Part print with two shaded views. Sizes in mm from the minimum x, y, z corner. A direction names the side the tool comes from. Round coordinates to 2 decimals unless told otherwise and drop trailing zeros. Write each loop counter-clockwise with the first axis right and the second up, starting at its lowest first coordinate (ties: lowest second). Pieces come first, ordered by that corner, then holes. Notation, with made-up numbers: (67, 36) -> (97, 36) arc R15 ccw to (97, 51) -> close; hole circle Ø10 at (74, 75). An arc over 180 degrees is marked (long way). Answer as CSV lines item,"result".
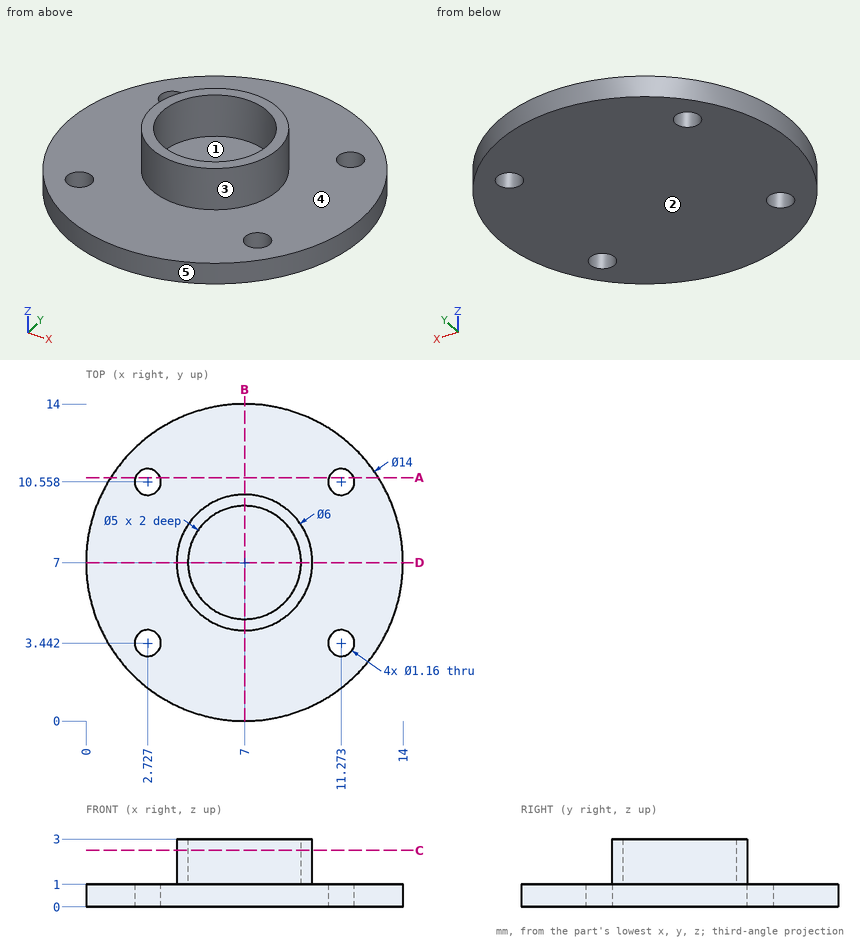
1. Cut at B-B, the plane x = 7. Write the cut outline in (y, z).
Results found:
outline,"(0, 0) -> (14, 0) -> (14, 1) -> (10, 1) -> (10, 3) -> (9.5, 3) -> (9.5, 1) -> (4.5, 1) -> (4.5, 3) -> (4, 3) -> (4, 1) -> (0, 1) -> close"
2. Mould opens along X. For the marked faces 1, 2 and 3 say: +X half, -X half, draft (parallel to the pull), parting line (faces both ways), or undercut.
Results found:
face 1,"undercut"
face 2,"draft"
face 3,"parting line"
3. Probe line 1 along Z through (x, y) = (8.75, 1.75); line 2 along Y through (x, z) = (7.5, 1.7); line 3 along Y through (x, z) = (7, 2.45). List the from-to ranges inside material, lowest first.
Results found:
line 1,"z = 0 to 1"
line 2,"y = 4.04 to 4.55, 9.45 to 9.96"
line 3,"y = 4 to 4.5, 9.5 to 10"
4. Cut at C-C, the plane z = 2.5. Write the cut outline in (x, y).
Results found:
outline,"circle Ø6 at (7, 7); hole circle Ø5 at (7, 7)"
5. Cut at A-A, the plane y = 10.75. Write the cut outline in (x, z) (1 decimal).
Results found:
outline,"(1.1, 0) -> (2.2, 0) -> (2.2, 1) -> (1.1, 1) -> close; (3.3, 0) -> (10.7, 0) -> (10.7, 1) -> (3.3, 1) -> close; (11.8, 0) -> (12.9, 0) -> (12.9, 1) -> (11.8, 1) -> close"
6. Which spindle directions (+Z, -Z, +X, -X, +Y, -Y) get a long thin tool onto all of the face, cutting with end or side? Do the marked faces 4 and 5. Say none if no direction does.
Results found:
face 4,"+Z"
face 5,"+Z, -Z"
7. Drop flat-ended pins along their axis: pin 1 Ø1.3 at (x, y) = (2.73, 3.44) entering from +Z; pin 2 Ø1 at (x, y) = (11.27, 3.44) entering from -Z; pin 3 Ø1.5 at (y, z) = (9.5, 0.5) entering from -X. Give the stop position or say it passes through.
Results found:
pin 1,"stops at z = 1"
pin 2,"passes through"
pin 3,"stops at x = 0.22"
